The model under review builds one solid part; all positions refer to its coordinate system, in mm. A direction names the side the tool comes from. Round coordinates to 2 decimals unless told otherwise and drop trailing zeros. Write each loop counter-clockwise with the first axis right and the second up, starting at its lowest first coordinate (ties: lowest second). Pieces come first, ordered by that corner, then holes. Notation, with made-up numbers: (23.5, -11.75) -> (39.5, -11.75) arc R10 cw to (39.5, 1.25) -> close; hole circle Ø10 at (16, 52.5). An arc over 180 degrees is marked (long way). Answer as a JSON object with one key per item and string values. Group by question number.
1) To check wall thickness, follow probe 1 along Y at (x, z) = (40.5, 40); probe 2 along Z at (x, y) = (57, -23.5); probe 3 along Z at (x, y) = (5, -98). State the ranges of each line that lie inside material, in increasing order. Write a range as [from, to].
2) We need section D-D, the plane x = 34.5. Write out the cut boundary in (y, z).
3) We need section B-B, the plane y = -16. Write out the cut boundary in (x, z), then the cut area to 3 significant figures.
4) Machinability: for faces 1 (the flat face through (62, -13, 0)), 2 (the flat face through (54, -13, 47.728)), 3 (the flat face through (77.761, -13, 24)), which of the approach directions +Z, -Z, +X, -X, +Y, -Y give a long, thin tool a straight path to every point of the face, cutting with its end or side? Answer none if there is none.
5) Insertion check: pin 1 Ø6 at (x, y) = (33, -108) entering from -Z; pin 2 Ø4 at (x, z) = (56, 14.5) entering from -Y; pin 3 Ø1 at (y, z) = (-91.5, 45.5) entering from -X. Each pin has a flat end and moves straight along its axis. Give the tip position at first contact, or say it passes through.
6) We need section C-C, the plane z = 41. Write out the cut boundary in (x, y).
7) We need section A-A, the plane x = 64. Write out the cut boundary in (y, z), then the cut area to 3 significant figures.
from build123d import *

# Parameters (mm, degrees)
F0_R      = 42.713148629
F1_DEPTH  = 66.9949576259
F1_FACE_R = 42.713148629
F2_W      = 52.3607060313
F2_H      = 47.7277636528
F3_DEPTH  = 25.4
F4_DEPTH  = 25.4
F5_DEPTH  = 25.4
F6_DEPTH  = 25.4


with BuildPart() as f1:
    # F0 (on Front) → F1 (new body)
    with BuildSketch(Plane.XZ):
        with Locations((6.7541077733, 13.033375144)):
            Circle(F0_R)
    extrude(amount=F1_DEPTH)

    # F1_face (on face) + F2 (on Front) → F3 (join)
    with BuildSketch(Plane(origin=(6.7541077733, -66.9949576259, 13.033375144), x_dir=(1, 0, 0), z_dir=(0, -1, 0))):
        Circle(F1_FACE_R)
    with BuildSketch(Plane.XZ):
        with Locations((26.1803530157, 23.8638818264)):
            Rectangle(F2_W, F2_H)
    extrude(amount=F3_DEPTH)

    # F4 (add): a face of the model
    f4_faces = [f1.faces().sort_by_distance(p)[0] for p in [
        (52.3607060313, -12.7, 23.8638818264),
    ]]
    extrude(f4_faces, amount=F4_DEPTH)

    # F5 (add): a face of the model
    f5_faces = [f1.faces().sort_by_distance(p)[0] for p in [
        (6.7541077733, -92.3949576259, 13.033375144),
    ]]
    extrude(f5_faces, amount=F5_DEPTH)

    # F6 (add): a face of the model
    f6_faces = [f1.faces().sort_by_distance(p)[0] for p in [
        (6.7541077733, -117.7949576259, 13.033375144),
    ]]
    extrude(f6_faces, amount=F6_DEPTH)


solid = f1.part
Here are the results:
{
 "1": {"probe 1": "y = [-25.4, 0]", "probe 2": "z = [0, 47.73]", "probe 3": "z = [-29.64, 55.71]"},
 "2": {"outline": "(-143.19, -19.44) -> (0, -19.44) -> (0, 47.73) -> (-25.4, 47.73) -> (-25.4, 45.51) -> (-143.19, 45.51) -> close"},
 "3": {"outline": "(31.67, 47.73) arc R42.71 ccw (long way) to (47.43, 0) -> (77.76, 0) -> (77.76, 47.73) -> close", "area": "7,280 mm^2"},
 "4": {"face 1": "-Z, +X, +Y, -Y", "face 2": "+Z, +X, +Y, -Y", "face 3": "+Z, -Z, +X, +Y, -Y"},
 "5": {"pin 1": "stops at z = -22.8", "pin 2": "stops at y = -25.4", "pin 3": "stops at x = -21.58"},
 "6": {"outline": "(-25.53, -143.19) -> (39.04, -143.19) -> (39.04, -25.4) -> (77.76, -25.4) -> (77.76, 0) -> (-25.53, 0) -> close"},
 "7": {"outline": "(-25.4, 0) -> (0, 0) -> (0, 47.73) -> (-25.4, 47.73) -> close", "area": "1,210 mm^2"}
}
